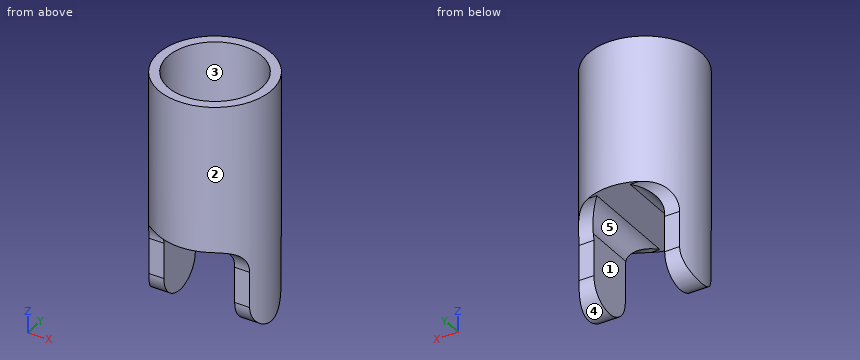
```python
from build123d import *

# Parameters (mm, degrees)
CUT_EXTRUDE1_DEPTH      = 38.432697939
CUT_EXTRUDE1_DEPTH_BACK = 38.432697939
CUT_EXTRUDE2_DEPTH      = 38.432698083
CUT_EXTRUDE2_DEPTH_BACK = 38.432698083


with BuildPart() as part:
    # Sketch1 → Revolve1 (revolve)
    with BuildSketch(Plane(origin=(0, 0, 0), x_dir=(0, 0, -1), z_dir=(1, 0, 0))):
        Polygon((-34.925, 9.525), (-34.925, 7.9375), (-15.925, 7.9375), (-15.925, 0), (9.525, 0), (9.525, 9.525), align=None)
    revolve(axis=Axis((0, 0, 0), (0, 0, 1)))

    # Sketch3 → Cut-Extrude1 (cut, two sides: drawn at the far end of the back side and taken through both)
    with BuildSketch(Plane(origin=(0, 0, 0), x_dir=(0, 0, -1), z_dir=(1, 0, 0)).offset(-CUT_EXTRUDE1_DEPTH_BACK)):
        with BuildLine():
            Line((9.525, 9.525), (-10.233333333, 9.525))
            Line((-10.233333333, 9.525), (-10.233333333, 8.466666667))
            ThreePointArc((-10.233333333, 8.466666667), (-8.993418707, 5.47324796), (-6, 4.233333333))
            Line((-6, 4.233333333), (0, 4.233333333))
            ThreePointArc((0, 4.233333333), (4.233333333, 0), (0, -4.233333333))
            Line((0, -4.233333333), (-6, -4.233333333))
            ThreePointArc((-6, -4.233333333), (-8.993418707, -5.47324796), (-10.233333333, -8.466666667))
            Line((-10.233333333, -8.466666667), (-10.233333333, -9.525))
            Line((-10.233333333, -9.525), (9.525, -9.525))
            Line((9.525, -9.525), (9.525, 9.525))
        make_face()
    extrude(amount=CUT_EXTRUDE1_DEPTH + CUT_EXTRUDE1_DEPTH_BACK, mode=Mode.SUBTRACT)

    # Sketch4 → Cut-Extrude2 (cut, two sides: drawn at the far end of the back side and taken through both)
    with BuildSketch(Plane(origin=(0, 0, 0), x_dir=(1, 0, 0), z_dir=(0, 1, 0)).offset(-CUT_EXTRUDE2_DEPTH_BACK)):
        with BuildLine():
            Line((-2.825, -10.233333333), (2.825, -10.233333333))
            ThreePointArc((2.825, -10.233333333), (5.07006403, -9.303397364), (6, -7.058333333))
            Line((6, -7.058333333), (6, 4.233333333))
            Line((6, 4.233333333), (-6, 4.233333333))
            Line((-6, 4.233333333), (-6, -7.058333333))
            ThreePointArc((-6, -7.058333333), (-5.07006403, -9.303397364), (-2.825, -10.233333333))
        make_face()
    extrude(amount=CUT_EXTRUDE2_DEPTH + CUT_EXTRUDE2_DEPTH_BACK, mode=Mode.SUBTRACT)


solid = part.part
```
For this review, take the finished solid that the model builds, in its own axes (mm). Face numbers are marked on the shaded views. A direction names the side the tool comes from. Give positions to 0.01 mm unless a question says otherwise; leave off trailing zeros. Order: outer loops, then holes, each group sorted by start corner. A loop starts at its lowest first (then second) coordinate and runs counter-clockwise, first axis right, second up.
1) Wall thickness on line 1 (X direction, y = 0, z = 21.5) (1 decimal); line 2 (Z direction, x = 0, y = 7) (3 decimals): over which ranges is each line inside the solid? List them lowest first.
2) For the marked faces 3, 4 and 5, list the 3-axis set-ups (+Z, -Z, +X, -X, +Y, -Y) from which the entire face can be reached by the end or side of a thin tool; tool diameter is ignored.
3) Insertion check: pin 1 (1 mm diameter, centred on x = -6, y = 4, fed in from -Z); pin 2 (1.5 mm diameter, centred on x = -6, y = -6, fed in from -Z); pin 3 (9.5 mm diameter, centred on x = 0, y = 0, fed in from -Z). Each pin has a flat end and moves straight along its axis. Give the tip position at first contact, or say it passes through.
4) Take a section at A-A (z = -1.5). Give the boundary of the cut face in (x, y) (3 decimals), then the cut area to 3 significant figures.
5) Take a section at B-B (x = 0). Give the boundary of the cut face in (y, z) (1 decimal), then the cut area to 3 significant figures.
6) The part is to be moulded in two halves that separate along X. For the marked faces 1 and 2, say which applies: released by +X, released by -X, zero draft, split by the parting line, or undercut.
Derived:
1. line 1: x = -9.5 to -7.9, 7.9 to 9.5
1. line 2: z = 10.233 to 15.925
2. face 3: +Z
2. face 4: -Z, +X, -X
2. face 5: -Z, +Y, -Y
3. pin 1: stops at z = -2.38
3. pin 2: stops at z = 8.75
3. pin 3: stops at z = 9.58
4. outline: (-8.663, -3.959) - (-6, -3.959) - (-6, 3.959) - (-8.663, 3.959) arc R9.525 ccw to start; (6, -3.959) - (8.663, -3.959) arc R9.525 ccw to (8.663, 3.959) - (6, 3.959) - close
4. area: 51.4 mm2
5. outline: (-9.5, 10.2) - (9.5, 10.2) - (9.5, 34.9) - (7.9, 34.9) - (7.9, 15.9) - (-7.9, 15.9) - (-7.9, 34.9) - (-9.5, 34.9) - close
5. area: 169 mm2
6. face 1: undercut
6. face 2: split by the parting line
